Build history of the part. All positions in model axes, mm. Face numbers are marked on the shaded views. Round coordinates to 2 decimals unless told otherwise and drop trailing zeros. Write each loop counter-clockwise with the first axis right and the second up, starting at its lowest first coordinate (ties: lowest second). Pieces come first, ordered by that corner, then holes.
Item 1: Band-saw the part on A-A, the plane y = 30. Count the separate pieces of the cut face and the enclosed holes in it, then the cut area to 3 significant figures.
Item 2: Wall check: probe 1 along Z at (x, y) = (-29.5, 19.5); probe 2 along X at (y, z) = (20, -4.5); probe 3 along Z at (x, y) = (-2.5, 25). Give the ranges that are in metal, low to high.
Item 3: Band-saw the part on C-C, the plane z = -35. Write the cut outline in (x, y).
Item 4: Mould opens along Y. For the marked faces 1, 2, 3 and 4 say: +Y half, -Y half, draft (parallel to the pull), parting line (faces both ways), or undercut.
Item 5: Band-saw the part on B-B, the plane x = -2.5. Write the cut outline in (y, z).
Item 6: Drop flat-ended pins along their axis: pin 1 Ø2.5 at (x, z) = (-2.5, -35) entering from -Y; pin 2 Ø1.6 at (x, z) = (-16, -12) entering from +Y; pin 3 Ø1.6 at (y, z) = (25.5, -20.5) entering from +X. Give the stop position or say it passes through.
Item 7: Band-saw the part on D-D, the plane x = -29.5. Write the cut outline in (y, z), then the cut area to 3 significant figures.
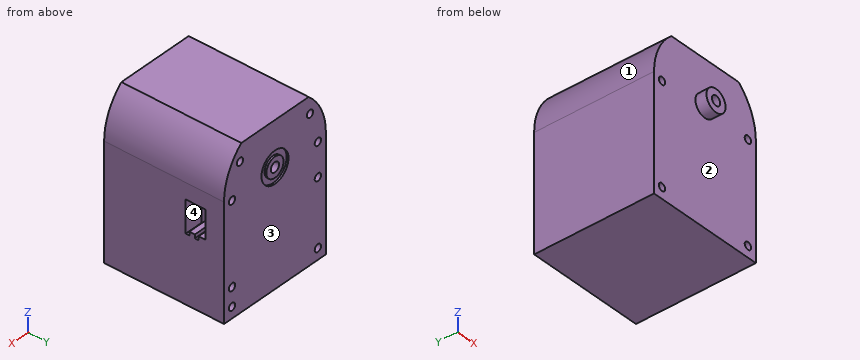
Autodesk Inventor part; units mm, degrees
ref_plane "YZ Plane" through (0, 0, 0) normal (1, 0, 0) x (0, 1, 0)
ref_plane "XZ Plane" through (0, 0, 0) normal (0, 1, 0) x (-1, 0, 0)
ref_plane "XY Plane" through (0, 0, 0) normal (0, 0, 1) x (1, 0, 0)
sketch "スケッチ1" plane through (0, 0, 0) normal (0, 1, 0) x (-1, 0, 0)
  line L0 (0, 0) -> (32, 0)
  line L1 (32, 0) -> (32, -43)
  line L2 (32, -43) -> (0, -43)
  line L3 (0, -43) -> (0, 0)
  dimension "d0" = 32
  dimension "d1" = 43
extrude "押し出し1" add sketch "スケッチ1" along normal blind 32.5
sketch "スケッチ2" plane through (0, 0, 0) normal (0, -1, 0) x (1, 0, 0)
  line L0 (-32, -43) -> (-32, 0) construction
  line L1 (-32, -21.5) -> (0, -21.5) construction
  line L2 (0, 0) -> (0, -43) construction
  line L3 (-16, -21.5) -> (-16, -12) construction
  line L4 (-32, 0) -> (-32, -43)
  arc A0 (-26.583, 0) -> (-32, -12) centre (-16, -12) ccw
  arc A1 (0, -12) -> (-5.417, 0) centre (-16, -12) ccw
  line L5 (-32, -12) -> (-32, 0)
  line L6 (0, 0) -> (-32, 0)
  line L7 (-5.417, 0) -> (0, 0)
  line L8 (0, 0) -> (0, -12)
  line L9 (-32, 0) -> (-26.583, 0)
  dimension "d4" = 9.5
extrude "押し出し2" cut sketch "スケッチ2" against normal blind 32.5
sketch "スケッチ3" plane through (0, 0, 0) normal (0, -1, 0) x (1, 0, 0)
  line L0 (-32, -21.5) -> (0, -21.5) construction
  line L1 (0, -21.5) -> (0, -43) construction
  line L2 (-5.417, 0) -> (-26.583, 0) construction
  line L3 (-16, 0) -> (-16, -43) construction
  line L4 (-32, -43) -> (0, -43) construction
  line L5 (-16, -21.5) -> (-16, -13) construction
  line L6 (-16, -21.5) -> (-29.5, -21.5) construction
  circle A0 centre (-29.5, -13) radius 1
  line L7 (-16, -21.5) -> (-2.5, -21.5) construction
  circle A1 centre (-2.5, -13) radius 1
  line L8 (-16, -21.5) -> (-16, -40) construction
  circle A2 centre (-29.5, -40) radius 1
  circle A3 centre (-2.5, -40) radius 1
  point P0 (0, 0)
  dimension "d8" = 8.5
  dimension "d9" = 13.5
  dimension "d10" = 2
  dimension "d11" = 13.5
  dimension "d12" = 2
  dimension "d13" = 18.5
  dimension "d14" = 2
  dimension "d15" = 2
extrude "押し出し3" cut sketch "スケッチ3" against normal blind 32.5
sketch "スケッチ4" plane through (0, 32.5, 0) normal (0, 1, 0) x (1, 0, 0)
  line L0 (-5.417, 0) -> (-26.583, 0) construction
  line L1 (-32, 21.5) -> (0, 21.5) construction
  line L2 (0, 21.5) -> (0, 43) construction
  line L3 (-16, 0) -> (-16, 43) construction
  line L4 (-32, 43) -> (0, 43) construction
  line L5 (-16, 21.5) -> (-16, 13) construction
  line L6 (-16, 21.5) -> (-29.5, 21.5) construction
  circle A0 centre (-29.5, 13) radius 1
  line L7 (-16, 21.5) -> (-2.5, 21.5) construction
  circle A1 centre (-2.5, 13) radius 1
  line L8 (-16, 21.5) -> (-16, 40) construction
  circle A2 centre (-29.5, 40) radius 1
  circle A3 centre (-2.5, 40) radius 1
  line L9 (-29.5, 21.5) -> (-29.5, 22) construction
  line L10 (-2.5, 21.5) -> (-2.5, 35) construction
  line L11 (-16, 21.5) -> (-16, 4.5) construction
  line L12 (-16, 4.5) -> (-5, 4.5) construction
  line L13 (-16, 4.5) -> (-27, 4.5) construction
  circle A4 centre (-2.5, 35) radius 1
  circle A5 centre (-29.5, 22) radius 1
  circle A6 centre (-27, 4.5) radius 1
  circle A7 centre (-5, 4.5) radius 1
  line L14 (0, 43) -> (-32, 43)
  line L15 (0, 43) -> (-32, 43)
  line L16 (-32, 43) -> (-32, 12)
  line L17 (-32, 43) -> (-32, 12)
  line L18 (0, 12) -> (0, 43)
  line L19 (0, 43) -> (0, 12)
  line L20 (-26.583, 0) -> (-5.417, 0)
  line L21 (-5.417, 0) -> (-26.583, 0)
  arc A8 (-32, 12) -> (-26.583, 0) centre (-16, 12) ccw
  arc A9 (-5.417, 0) -> (0, 12) centre (-16, 12) ccw
  arc A10 (-5.417, 0) -> (0, 12) centre (-16, 12) ccw
  point P0 (0, 0)
  point P1 (0, 0)
  dimension "d26" = 0.5
  dimension "d27" = 13.5
  dimension "d28" = 17
  dimension "d29" = 11
  dimension "d30" = 11
  dimension "d31" = 2
  dimension "d32" = 2
  dimension "d33" = 2
  dimension "d34" = 2
extrude "押し出し4" cut sketch "スケッチ4" against normal blind 30 contours A4 | A5 | A6 | A7
sketch "スケッチ5" plane through (0, 0, 0) normal (0, -1, 0) x (1, 0, 0)
  line L0 (-32, -21.5) -> (0, -21.5) construction
  line L1 (0, -21.5) -> (0, -43) construction
  line L2 (-5.417, 0) -> (-26.583, 0) construction
  line L3 (-16, 0) -> (-16, -43) construction
  line L4 (-32, -43) -> (0, -43) construction
  line L5 (-16, -21.5) -> (-16, -12) construction
  line L6 (-16, -21.5) -> (-29.5, -21.5) construction
  circle A0 centre (-29.5, -13) radius 1
  line L7 (-16, -21.5) -> (-2.5, -21.5) construction
  circle A1 centre (-2.5, -13) radius 1
  line L8 (-16, -21.5) -> (-16, -40) construction
  circle A2 centre (-29.5, -40) radius 1
  circle A3 centre (-2.5, -40) radius 1
  circle A4 centre (-16, -12) radius 3
  point P0 (0, 0)
  point P1 (0, 0)
  dimension "d37" = 9.5
  dimension "d38" = 13.5
  dimension "d39" = 2
  dimension "d40" = 13.5
  dimension "d41" = 2
  dimension "d42" = 18.5
  dimension "d43" = 2
  dimension "d44" = 2
  dimension "d45" = 6
extrude "押し出し5" add sketch "スケッチ5" along normal blind 3 contours A4
sketch "スケッチ6" plane through (-16, -3, -12) normal (0, -1, 0) x (1, 0, 0)
  circle A0 centre (0, 0) radius 1.3
  point P0 (16, 12)
  dimension "d48" = 2.6
extrude "押し出し6" cut sketch "スケッチ6" against normal blind 7
sketch "スケッチ7" plane through (0, 32.5, 0) normal (0, 1, 0) x (1, 0, 0)
  line L0 (-5.417, 0) -> (-26.583, 0) construction
  line L1 (-16, 21.5) -> (-29.5, 21.5) construction
  line L2 (-16, 21.5) -> (-16, 13) construction
  line L3 (-16, 21.5) -> (-2.5, 21.5) construction
  line L4 (-32, 21.5) -> (0, 21.5) construction
  line L5 (-32, 43) -> (0, 43) construction
  line L6 (-16, 21.5) -> (-16, 40) construction
  line L7 (0, 21.5) -> (0, 43) construction
  line L8 (-16, 0) -> (-16, 43) construction
  line L9 (-29.5, 21.5) -> (-29.5, 22) construction
  line L10 (-16, 21.5) -> (-16, 12) construction
  line L11 (-16, 12) -> (-5, 12) construction
  line L12 (-16, 12) -> (-27, 12) construction
  circle A0 centre (-16, 12) radius 1.3
  circle A1 centre (-16, 12) radius 4.25
  point P0 (0, 0)
  point P1 (0, 0)
  point P2 (0, 0)
  dimension "d53" = 9.5
  dimension "d60" = 8.5
extrude "押し出し7" cut sketch "スケッチ7" against normal blind 0.5 contours A0 | A1
sketch "スケッチ8" plane through (-16, 32, -12) normal (0, 1, 0) x (1, 0, 0)
  circle A0 centre (0, 0) radius 2.7
  point P0 (16, -12)
  dimension "d63" = 5.4
extrude "押し出し8" add sketch "スケッチ8" along normal blind 0.5
sketch "スケッチ9" plane through (-16, 32.5, -12) normal (0, 1, 0) x (1, 0, 0)
  circle A0 centre (0, 0) radius 1.3
  point P0 (16, -12)
  dimension "d66" = 2.6
extrude "押し出し9" cut sketch "スケッチ9" against normal blind 10
sketch "スケッチ10" plane through (0, 0, -43) normal (1, 0, 0) x (0, 0, -1)
  line L0 (0, 0) -> (0, 32.5) construction
  line L1 (0, 16.25) -> (-21.5, 16.25) construction
  line L2 (-22, 32.5) -> (-20, 32.5) construction
  line L3 (0, 0) -> (-31, 0) construction
  line L4 (-21, 32.5) -> (-21, 27.5) construction
  line L5 (-21, 27.5) -> (-26.7, 27.5)
  line L6 (-26.7, 27.5) -> (-26.7, 24.6)
  line L7 (-26.7, 24.6) -> (-18, 24.6)
  line L8 (-18, 24.6) -> (-18, 25.6)
  line L9 (-18, 25.6) -> (-19, 25.6)
  line L10 (-19, 25.6) -> (-19, 27.5)
  line L11 (-19, 27.5) -> (-21, 27.5)
  line L12 (-26.7, 24.6) -> (-26.7, 22.1)
  line L13 (-26.7, 22.1) -> (-18, 22.1)
  line L14 (-18, 22.1) -> (-18, 23.1)
  line L15 (-18, 23.1) -> (-19, 23.1)
  line L16 (-19, 23.1) -> (-19, 24.6)
  point P0 (-43, 0)
  dimension "d69" = 21.5
  dimension "d71" = 5
  dimension "d72" = 2.9
  dimension "d73" = 5.7
  dimension "d74" = 8.7
  dimension "d75" = 1
  dimension "d76" = 1
  dimension "d79" = 2.5
  dimension "d80" = 1
  dimension "d81" = 1
extrude "押し出し10" cut sketch "スケッチ10" against normal blind 5
properties part number "Servo" material "プラスチック、不透明 黒"
Results:
1. separate pieces: 1
1. enclosed holes: 9
1. area: 1,310 mm2
2. probe 1: z = -43 to -41, -39 to -23, -21 to -14, -12 to -3.41
2. probe 2: x = -30.13 to -28, -26 to -6, -4 to -1.87
2. probe 3: z = -43 to -41, -39 to -36, -34 to -25, -16.3 to -14, -12 to -3.41
3. outline: (-32, 0) - (0, 0) - (0, 32.5) - (-1.5, 32.5) - (-1.5, 2.5) - (-3.5, 2.5) - (-3.5, 32.5) - (-32, 32.5) - close
4. face 1: draft
4. face 2: -Y half
4. face 3: +Y half
4. face 4: undercut
5. outline: (0, -43) - (32.5, -43) - (32.5, -41) - (0, -41) - close; (0, -39) - (32.5, -39) - (32.5, -36) - (2.5, -36) - (2.5, -34) - (32.5, -34) - (32.5, -14) - (0, -14) - close; (0, -12) - (32.5, -12) - (32.5, -3.41) - (0, -3.41) - close; hole (22.1, -25) - (23.1, -25) - (23.1, -24) - (24.6, -24) - (24.6, -25) - (25.6, -25) - (25.6, -24) - (27.5, -24) - (27.5, -16.3) - (22.1, -16.3) - close
6. pin 1: stops at y = 0
6. pin 2: stops at y = 22.5
6. pin 3: stops at x = -5
7. outline: (0, -43) - (32.5, -43) - (32.5, -41) - (0, -41) - close; (0, -39) - (32.5, -39) - (32.5, -23) - (2.5, -23) - (2.5, -21) - (32.5, -21) - (32.5, -14) - (0, -14) - close; (0, -12) - (32.5, -12) - (32.5, -3.41) - (0, -3.41) - close
7. area: 1,100 mm2
